```python
from build123d import *

# Parameters (mm, degrees)
F0_W          = 274.5
F0_H          = 10
F1_DEPTH      = 175.5
F2_T          = -2.5
F3_R          = 2
F4_DEPTH      = 10
F4_DEPTH_BACK = 185
F5_W          = 27.900162
F5_H          = 2.426103
F6_DEPTH      = 15
F7_R          = 3.313437
F8_DEPTH      = 25


with BuildPart() as f1:
    # F0 (on Top) → F1 (new body)
    with BuildSketch(Plane.XY):
        with Locations((137.25, 5)):
            Rectangle(F0_W, F0_H)
    extrude(amount=F1_DEPTH)

    # F2
    f2_openings = [f1.faces().sort_by_distance(p)[0] for p in [
        (137.25, 10, 87.75),
    ]]
    offset(amount=F2_T, openings=f2_openings)

    # F3 (on face) → F4 (join, two sides)
    with BuildSketch(Plane(origin=(0, 0, 0), x_dir=(1, 0, 0), z_dir=(0, 0, -1))) as f4_sk:
        with Locations((265.5, -5)):
            Circle(F3_R)
    extrude(amount=F4_DEPTH)
    extrude(f4_sk.sketch, amount=-F4_DEPTH_BACK)

    # F5 (on face) → F6 (join)
    with BuildSketch(Plane.XZ):
        with Locations((22.99581, 110.854611)):
            Rectangle(F5_W, F5_H)
    extrude(amount=F6_DEPTH)

    # F7 (on face) → F8 (cut)
    with BuildSketch(Plane(origin=(0, 0, 109.641559), x_dir=(1, 0, 0), z_dir=(0, 0, -1))):
        with Locations((22.99581, 7.5)):
            Circle(F7_R)
    extrude(amount=-F8_DEPTH, mode=Mode.SUBTRACT)


solid = f1.part
```
CAD build for the part. Positions are in the model's coordinates, mm. A direction names the side the tool comes from. Round coordinates to 2 decimals unless told otherwise and drop trailing zeros. Write each loop counter-clockwise with the first axis right and the second up, starting at its lowest first coordinate (ties: lowest second). Pieces come first, ordered by that corner, then holes. Notation, with made-up numbers: (46.25, 58) - (79.25, 58) arc R15 cw to (79.25, 66) - close; hole circle Ø4 at (43, -38.75). An arc over 180 degrees is marked (long way). Return JSON: item names as keys, results as strings. Group by question number.
Item 1: Band-saw the part on B-B on y = -7.5. List the corners of the cut face in (x, z), plus the area to 3 significant figures.
Item 2: 3-axis set-ups, long thin cutter, end or side, ignore diameter. For faces 1 (the face through (2.5, 6, 87)), 2 (the face through (23, -4, 112.068)), 3 (the face through (23, -4, 109.642)): which of +Z, -Z, +X, -X, +Y, -Y reach the whole face in a straight line?
Item 3: Mould opens along X. For faces 4 (the face through (0, 5, 87)), 5 (the face through (135, 6, 173)), 6 (the face through (135, 0, 87)) say: +X half, -X half, draft (parallel to the pull), parting line (faces both ways), or undercut.
Item 4: Probe probe 1 along X at (y, z) = (5, 5.5); probe 2 along X at (y, z) = (7.25, 166); probe 3 along X at (y, z) = (-7.5, 110.45). List the from-to ranges inside material, lowest first.
Item 5: Band-saw the part on A-A on z = 36.5. List the corners of the cut face in (x, y), plus the area to 3 significant figures.
Item 6: Flat gauge pins, fed straight in: pin 1 Ø5 at (y, z) = (1.5, 155) entering from -X; pin 2 Ø3 at (x, z) = (191, 42) entering from +Y; pin 3 Ø6 at (x, z) = (36.5, 88) entering from -Y; pin 4 Ø7.5 at (x, y) = (23, -7.5) entering from +Z. Where does each tip first touch, or does it go through?
Item 7: Band-saw the part on C-C on x = 90. List the corners of the cut face in (y, z), plus the area to 3 significant figures.
Resolved:
{
 "1": {"outline": "(9.05, 109.64) - (19.68, 109.64) - (19.68, 112.07) - (9.05, 112.07) - close; (26.31, 109.64) - (36.95, 109.64) - (36.95, 112.07) - (26.31, 112.07) - close", "area": "51.6 mm²"},
 "2": {"face 1": "+Y", "face 2": "+Z, +X, -X, -Y", "face 3": "-Z, +X, -X, -Y"},
 "3": {"face 4": "-X half", "face 5": "undercut", "face 6": "draft"},
 "4": {"probe 1": "x = 0 to 2.5, 263.5 to 267.5, 272 to 274.5", "probe 2": "x = 0 to 2.5, 272 to 274.5", "probe 3": "x = 9.05 to 19.68, 26.31 to 36.95"},
 "5": {"outline": "(0, 0) - (274.5, 0) - (274.5, 10) - (272, 10) - (272, 2.5) - (2.5, 2.5) - (2.5, 10) - (0, 10) - close; circle Ø4 at (265.5, 5)", "area": "736 mm²"},
 "6": {"pin 1": "stops at x = 0", "pin 2": "stops at y = 2.5", "pin 3": "stops at y = 0", "pin 4": "stops at z = 112.07"},
 "7": {"outline": "(0, 0) - (10, 0) - (10, 2.5) - (2.5, 2.5) - (2.5, 173) - (10, 173) - (10, 175.5) - (0, 175.5) - close", "area": "476 mm²"}
}
